Geometry check sheet. Reference: drawing and pictorial views, mm from the part's lowest x, y, z. Round coordinates to 2 decimals unless told otherwise and drop trailing zeros. Write each loop counter-clockwise with the first axis right and the second up, starting at its lowest first coordinate (ties: lowest second). Pieces come first, ordered by that corner, then holes. Notation, with made-up numbers: (-22.75, -17) - (34.25, -17) arc R6 ccw to (34.25, -13) - close; hole circle Ø3 at (1.25, 43.5). An arc over 180 degrees is marked (long way). Return JSON: item names as keys, results as strings.
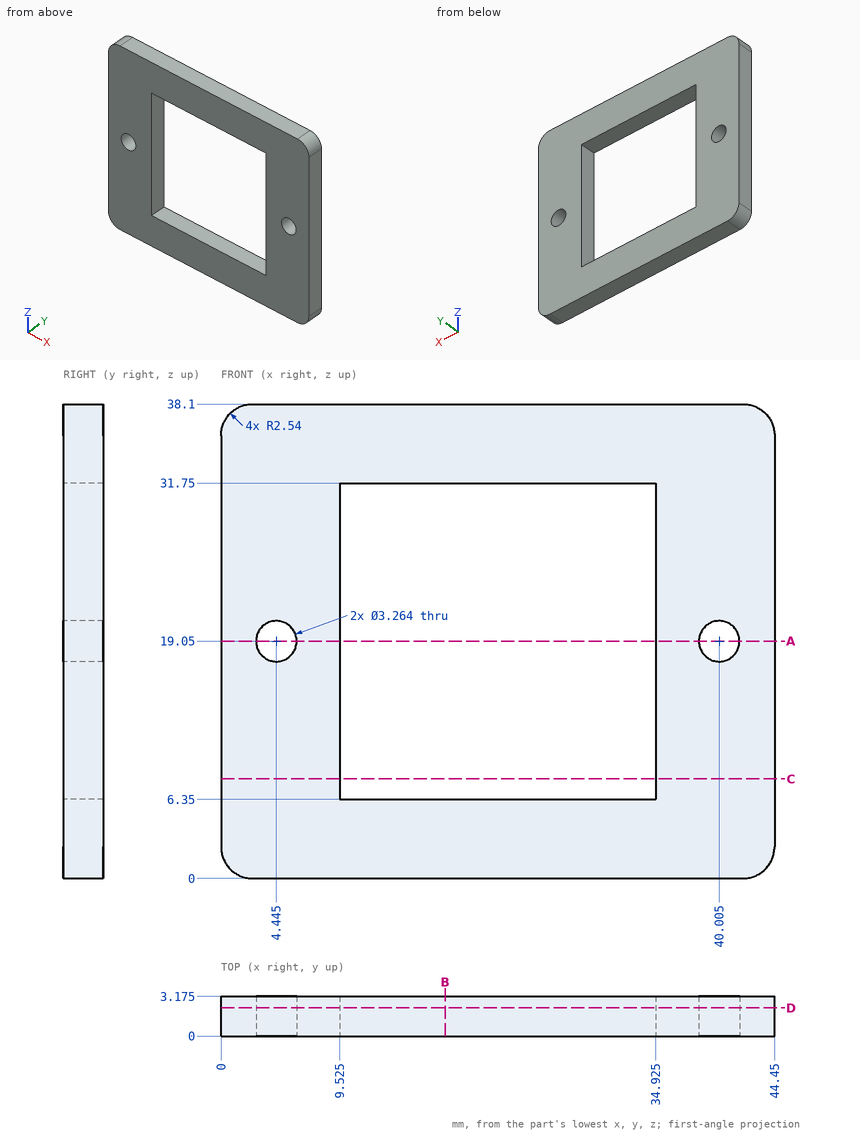
(1) Section check D-D, the plane y = 2.25. Enter the section's corners in (x, z) (3 decimals).
Response values:
{"outline": "(0, 2.54) arc R2.54 ccw to (2.54, 0) - (41.91, 0) arc R2.54 ccw to (44.45, 2.54) - (44.45, 35.56) arc R2.54 ccw to (41.91, 38.1) - (2.54, 38.1) arc R2.54 ccw to (0, 35.56) - close; hole circle Ø3.264 at (4.445, 19.05); hole (9.525, 6.35) - (34.925, 6.35) - (34.925, 31.75) - (9.525, 31.75) - close; hole circle Ø3.264 at (40.005, 19.05)"}
(2) Section check A-A, the plane z = 19.05. Enter the section's corners in (x, y) (3 decimals).
Response values:
{"outline": "(0, 0) - (2.813, 0) - (2.813, 3.175) - (0, 3.175) - close; (6.077, 0) - (9.525, 0) - (9.525, 3.175) - (6.077, 3.175) - close; (34.925, 0) - (38.373, 0) - (38.373, 3.175) - (34.925, 3.175) - close; (41.637, 0) - (44.45, 0) - (44.45, 3.175) - (41.637, 3.175) - close"}
(3) Section check C-C, the plane z = 8. Enter the section's corners in (x, y) (3 decimals).
Response values:
{"outline": "(0, 0) - (9.525, 0) - (9.525, 3.175) - (0, 3.175) - close; (34.925, 0) - (44.45, 0) - (44.45, 3.175) - (34.925, 3.175) - close"}
(4) Material ranges on line 1 along X through (y, z) = (1.9, 19.05) (3 decimals); line 2 along Z through (x, y) = (10, 0.3); line 3 along X through (y, z) = (2.3, 25) (3 decimals), recorded low to high. Write a range as [from, to].
Response values:
{"line 1": "x = [0, 2.813], [6.077, 9.525], [34.925, 38.373], [41.637, 44.45]", "line 2": "z = [0, 6.35], [31.75, 38.1]", "line 3": "x = [0, 9.525], [34.925, 44.45]"}
(5) Section check B-B, the plane x = 18. Enter the section's corners in (y, z) (3 decimals).
Response values:
{"outline": "(0, 0) - (3.175, 0) - (3.175, 6.35) - (0, 6.35) - close; (0, 31.75) - (3.175, 31.75) - (3.175, 38.1) - (0, 38.1) - close"}
(6) Gauge pin test, flat end, axial feed: pin 1 (3 mm diameter, centred on x = 4.445, z = 19.05, fed in from -Y). Record the tip position at first contact, or that the pin passes through.
Response values:
{"pin 1": "passes through"}
